Verification items for the finished model (mm, model axes). Coordinates: 2 decimals unless noted, no trailing zeros. Order: outer loops, then holes, each group sorted by start corner. A loop starts at its lowest first (then second) coordinate and runs counter-clockwise, first axis right, second up.
Q1. Cross-section at A-A, the plane z = 47. Record the boundary of the cut face in (x, y).
Q2. Cross-section at C-C, the plane z = 35.5. Record the boundary of the cut face in (x, y), and give its area (3 significant figures).
Q3. Draft check along Y on faces 1 (the flat face through (0, 0, -51.554)), 2 (the conical face through (-7.109, 32.013, -0.872)), 3 (the conical face through (-14.23, 34.33, -9.88)). Enter one of: pulls with the +Y half, pulls with the -Y half, needs draft (parallel to the pull), parting line crosses it, or undercut.
Q4. Depth check by flat-ended pin: P1, Ø4, axis at x = -18, z = 38, coming from the +Y side; P2, Ø22, axis at x = 6.5, y = 5.5, coming from the +Z side; P3, Ø5, axis at y = 3, z = 15.5, coming from the +X side. Enter the tip coordinate at first touch or a pass-through.
Q5. Thickness scan on line 1 (Z direction, x = 1, y = 5); line 2 (Y direction, x = 24, z = 20); line 3 (X direction, y = 15, z = 8). Record the ranges inside material, lowest first.
Q6. Cross-section at B-B, the plane z = -38. Record the boundary of the cut face in (x, y), and give its area (3 significant figures).
from build123d import *

# Parameters (mm, degrees)
F2_R = 5.08


# Not quite as in the source:
# - a fillet or chamfer that OpenCascade refuses, or shapes differently, is made with other operations: its cross-section is extruded or revolved along the edge and cut away or added


with BuildPart() as f1:
    # F0 (on Right) → F1 (revolve)
    with BuildSketch(Plane.YZ):
        Polygon((31.2051475048, 40.8137366176), (0, 38.317322731), (0, -51.5535026789), (23.7159132957, -51.5535026789), (64.1577839851, 73.7663730979), align=None)
    revolve(axis=Axis((0, 0, -6.6180899739), (0, 0, -1)))

    # F2
    f2_edges = [f1.edges().sort_by_distance(p)[0] for p in [
        (0, -64.157784, 73.766373),
    ]]
    fillet(f2_edges, radius=F2_R)

    # F3 (on Front) → F4 (revolve, cut)
    with BuildSketch(Plane.XZ):
        Polygon((48.9296764135, 49.8008169234), (0, 49.8008169234), (0, -34.0786203742), (22.218067199, -34.0786203742), align=None)
    revolve(axis=Axis((0, 0, 7.8610982746), (0, 0, -1)), mode=Mode.SUBTRACT)

    # F5: fillet of radius 5.08 on 1 edges, made by hand

    # F5_s1 → F5_t2 (revolve, cut)
    with BuildSketch(Plane.YZ):
        with BuildLine():
            ThreePointArc((48.0680960352, 57.6766851479), (46.6103251908, 53.5321519556), (48.9296764135, 49.8008169234))
            Line((48.9296764135, 49.8008169234), (48.8750659721, 49.7151416079))
            ThreePointArc((48.8750659721, 49.7151416079), (44.5609521121, 49.6992169234), (40.1922278106, 49.6992169234))
            Line((40.1922278106, 49.6992169234), (40.1203857617, 49.8726589723))
            Line((40.1203857617, 49.8726589723), (47.9962539862, 57.7485271969))
            Line((47.9962539862, 57.7485271969), (48.0680960352, 57.6766851479))
        make_face()
    revolve(axis=Axis((0, 0, 49.8008169234), (0, 0, -1)), mode=Mode.SUBTRACT)


solid = f1.part
Check values:
1. outline: circle Ø111.04 at (0, 0); hole circle Ø96.08 at (0, 0)
2. outline: circle Ø103.62 at (0, 0); hole circle Ø88.75 at (0, 0)
2. area: 2,250 mm2
3. face 1: needs draft
3. face 2: undercut
3. face 3: parting line crosses it
4. P1: stops at y = 50.41
4. P2: stops at z = -34.08
4. P3: stops at x = 46.08
5. line 1: z = -51.55 to -34.08
5. line 2: y = -40.19 to -31.3, 31.3 to 40.19
5. line 3: x = -40.23 to -32.31, 32.31 to 40.23
6. outline: circle Ø56.18 at (0, 0)
6. area: 2,480 mm2
